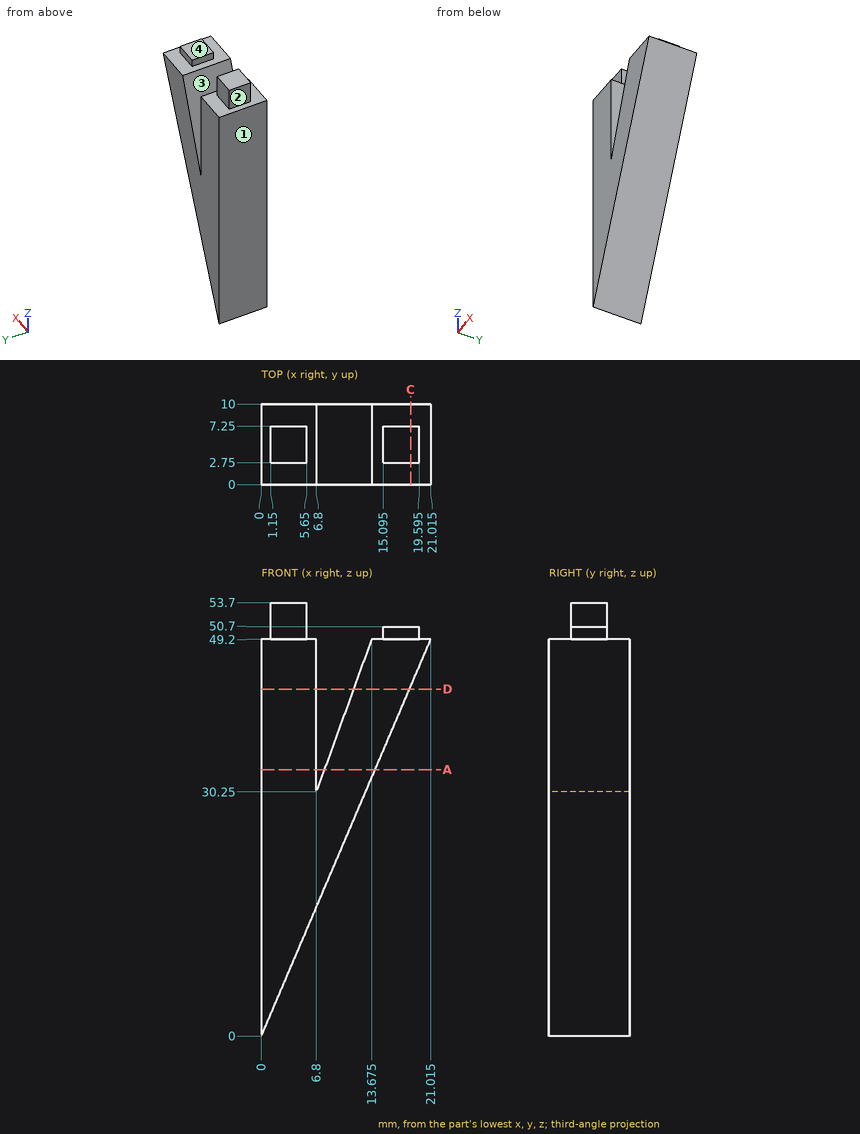
Print and shaded views of the part. All mm, measured from the part's lowest x, y and z. A direction names the side the tool comes from. Give positions to 0.01 mm unless a question says otherwise; leave off trailing zeros. Order: outer loops, then holes, each group sorted by start corner. A loop starts at its lowest first (then second) coordinate and runs counter-clockwise, first axis right, second up. Notation, with made-up numbers: (41, 74) -> (83, 74) arc R10 ccw to (83, 87) -> close; hole circle Ø11 at (-18.75, 69). An arc over 180 degrees is marked (long way). Use CSV: the item, a comma, the result in double quotes.
1. 3-axis set-ups, long thin cutter, end or side, ignore diameter. For the marked faces 1, 2, 3 and 4: which of +Z, -Z, +X, -X, +Y, -Y reach the whole face in a straight line?
Outcome:
face 1,"+Z, -Z, -X, +Y, -Y"
face 2,"+Z, -X, +Y, -Y"
face 3,"+Z, +Y, -Y"
face 4,"+Z, +X, +Y, -Y"
2. Band-saw the part on A-A, the plane z = 33. Give the cut face in (x, y) (1 decimal), then the cut area to 3 significant figures.
Outcome:
outline,"(0, 0) -> (6.8, 0) -> (6.8, 10) -> (0, 10) -> close; (7.8, 0) -> (14.1, 0) -> (14.1, 10) -> (7.8, 10) -> close"
area,"131 mm²"
3. Band-saw the part on D-D, the plane z = 43. Give the cut face in (x, y) (1 decimal).
Outcome:
outline,"(0, 0) -> (6.8, 0) -> (6.8, 10) -> (0, 10) -> close; (11.4, 0) -> (18.4, 0) -> (18.4, 10) -> (11.4, 10) -> close"
4. Drill centre lines: line 1 along X through (y, z) = (6.25, 31); line 2 along X through (y, z) = (8.75, 32) (1 decimal); line 3 along X through (y, z) = (3, 29) (1 decimal). Where is each one in solid material? Low to high. Write a range as from..to.
Outcome:
line 1,"0..6.8, 7.07..13.24"
line 2,"0..6.8, 7.4..13.7"
line 3,"0..12.4"
5. Drop flat-ended pins along their axis: pin 1 (1.3 mm diameter, centred on x = 4.5, z = 52, fed in from -Y); pin 2 (0.8 mm diameter, centred on y = 5.5, z = 50, fed in from -X); pin 3 (2 mm diameter, centred on x = 18.5, y = 4, fed in from +Z). Give the stop position or say it passes through.
Outcome:
pin 1,"y = 2.75"
pin 2,"x = 1.15"
pin 3,"z = 50.7"
6. Band-saw the part on C-C, the plane x = 18.5. Give the cut face in (y, z).
Outcome:
outline,"(0, 43.31) -> (10, 43.31) -> (10, 49.2) -> (7.25, 49.2) -> (7.25, 50.7) -> (2.75, 50.7) -> (2.75, 49.2) -> (0, 49.2) -> close"
